Verification items for the finished model (mm, model axes). A direction names the side the tool comes from. Coordinates: 2 decimals unless noted, no trailing zeros. Order: outer loops, then holes, each group sorted by start corner. A loop starts at its lowest first (then second) coordinate and runs counter-clockwise, first axis right, second up. Notation, with made-up numbers: M 48,18 L 66,18 A22 cw 66,48 Z; hole C -20.75,12 d10. An arc over 180 degrees is marked long. Return JSON: item names as keys, results as strings.
```python
from build123d import *

# Parameters (mm, degrees)
CHAMFER_1_SIZE  = 4
CHAMFER_1_SIZE2 = 2.309401077


with BuildPart() as part:
    # Эскиз1 → Повернуть1 (revolve)
    with BuildSketch(Plane.XY, mode=Mode.PRIVATE) as revolve_1_sk:
        Polygon((13.5, 0), (44.5, 0), (44.5, 3), (41, 8), (41, 10), (13.5, 10), align=None)
    revolve(revolve_1_sk.sketch.rotate(Axis((0, 0, 0), (0, 1, 0)), 90), axis=Axis((0, 0, 0), (0, 1, 0)))

    # Фаска1
    chamfer_1_edges = [part.edges().sort_by_distance(p)[0] for p in [
        (0, 0, 13.5),
    ]]
    chamfer_1_side = [part.faces().sort_by_distance(p)[0] for p in [
        (0, 0, 14.758650071),
    ]]
    chamfer(chamfer_1_edges, length=CHAMFER_1_SIZE, length2=CHAMFER_1_SIZE2, reference=chamfer_1_side[0])


solid = part.part
```
Q1. Material ranges on line 1 along X through (y, z) = (8, 0); line 2 along X through (y, z) = (4.5, 0); line 3 along Y through (x, z) = (39, -17.5), recorded low to high.
Values:
{"line 1": "-41 to -13.5, 13.5 to 41", "line 2": "-43.45 to -13.5, 13.5 to 43.45", "line 3": "0 to 5.51"}
Q2. Go/stop test with flat-tipped pins: pin 1 (2 mm diameter, centred on x = -11.5, y = 5.5, fed in from +Z); pin 2 (2 mm diameter, centred on y = 1.5, z = 5.5, fed in from -X); pin 3 (2 mm diameter, centred on x = -28, y = 3, fed in from +Z). Record where each tip stops, or that it passes through.
Values:
{"pin 1": "z = 41.95", "pin 2": "x = -44.27", "pin 3": "z = 35.37"}
Q3. Tool access check on faces 1 (the face through (15.703, 9.014, -37.874)), 2 (the face through (-1, 0, 19)). Record the directions out of +Z, -Z, +X, -X, +Y, -Y that give a thin tool (end or side, any length) a straight path to the whole face; none if there is none.
Values:
{"face 1": "+Y", "face 2": "+Z, -Z, +X, -X, -Y"}
Q4. Cross-section at A-A, the plane x = 0. Record the boundary of the cut face in (y, z), and give its area (3 significant figures).
Values:
{"outline": "M 0,-44.5 L 3,-44.5 L 8,-41 L 10,-41 L 10,-13.5 L 2.31,-13.5 L 0,-17.5 Z; M 0,17.5 L 2.31,13.5 L 10,13.5 L 10,41 L 8,41 L 3,44.5 L 0,44.5 Z", "area": "579 mm^2"}
Q5. Draft check along Z on faces 3 (the face through (-10, 10, 10)), 4 (the face through (13.18, 6.1, 2.93)), 5 (the face through (-30.075, 1.521, 32.798)). Enter one of: pulls with the +Z half, pulls with the -Z half, needs draft (parallel to the pull), parting line crosses it, or undercut.
Values:
{"face 3": "needs draft", "face 4": "undercut", "face 5": "parting line crosses it"}
Q6. Cross-section at B-B, the plane z = 0. Record the boundary of the cut face in (x, y).
Values:
{"outline": "M -44.5,0 L -17.5,0 L -13.5,2.31 L -13.5,10 L -41,10 L -41,8 L -44.5,3 Z; M 13.5,2.31 L 17.5,0 L 44.5,0 L 44.5,3 L 41,8 L 41,10 L 13.5,10 Z"}
